Here's how the part is built. I have some questions about the finished solid (model axes, mm). A direction names the side the tool comes from. Coordinates: 2 decimals unless noted, no trailing zeros. Write each loop counter-clockwise with the first axis right and the second up, starting at its lowest first coordinate (ties: lowest second). Pieces come first, ordered by that corner, then holes.
```python
from build123d import *

# Parameters (mm, degrees)
F0_R            = 22
F1_DEPTH        = 5
F3_DEPTH        = 25
F3_COPIES_COUNT = 8
F5_DEPTH        = 8
F5_COPIES_COUNT = 4


# Not quite as in the source:
# - a pattern or mirror of a feature is missing from the dataset's text; its kind, count and spacing are read off the source's solid
# - a feature names something its author has since deleted; it is built from what else it names


with BuildPart() as f1:
    # F0 (on Front) → F1 (new body)
    with BuildSketch(Plane.XZ):
        Circle(F0_R)
    extrude(amount=F1_DEPTH)

    # F2 (on face) → F3 (cut)
    with BuildSketch(Plane.XZ.offset(5)):
        with BuildLine():
            ThreePointArc((0, -9.25), (-1.9445436483, -13.9445436483), (2.75, -12))
            ThreePointArc((2.75, -12), (1.9445436483, -10.0554563517), (0, -9.25))
        make_face()
    f3 = extrude(amount=-F3_DEPTH, mode=Mode.SUBTRACT)

    # F3_copies: F3 ×8 about axis
    f3_copies_axis = Axis((0, 0, 0), (0, 1, 0))
    for i in range(1, F3_COPIES_COUNT):
        add(f3.rotate(f3_copies_axis, i * 360 / F3_COPIES_COUNT), mode=Mode.SUBTRACT)

    # F4 (on face) → F5 (join)
    with BuildSketch(Plane(origin=(0, 0, 0), x_dir=(-1, 0, 0), z_dir=(0, 1, 0))):
        with BuildLine():
            ThreePointArc((-5.7402514855, 13.8581929877), (-4.3938929457, 14.9631208861), (-3.8883017826, 16.6298315852))
            ThreePointArc((-3.8883017826, 16.6298315852), (-9.3827106195, 18.2965422843), (-5.7402514855, 13.8581929877))
        make_face()
    f5 = extrude(amount=F5_DEPTH)

    # F5_copies: F5 ×4 about axis
    f5_copies_axis = Axis((0, 0, 0), (0, 1, 0))
    for i in range(1, F5_COPIES_COUNT):
        add(f5.rotate(f5_copies_axis, i * 360 / F5_COPIES_COUNT))


solid = f1.part
```
1) Imagine slicing it at A-A on y = 1.5. Please give me the cut outline in (x, z).
Values follow:
outline: circle Ø6 at (-16.63, 6.89); circle Ø6 at (-6.89, -16.63); circle Ø6 at (6.89, 16.63); circle Ø6 at (16.63, -6.89)
2) Will these pins go through, and if not, where does the flat tip stop? pin 1 (7 mm diameter, centred on x = 12, z = 0, fed in from -Y); pin 2 (5 mm diameter, centred on y = 0, z = 14.5, fed in from +X); pin 3 (2 mm diameter, centred on y = -1, z = 10.5, fed in from +X); pin 4 (6.5 mm diameter, centred on x = 0, z = 12, fed in from +Y).
Values follow:
pin 1: stops at y = -5
pin 2: stops at x = 18.44
pin 3: stops at x = 19.84
pin 4: stops at y = 0
3) Imagine slicing it at C-C on x = -16. Please give me the cut outline in (y, z), then the cut area to 3 significant figures.
Values follow:
outline: (-5, -15.1) - (0, -15.1) - (0, 3.96) - (8, 3.96) - (8, 9.82) - (0, 9.82) - (0, 15.1) - (-5, 15.1) - close
area: 198 mm2
4) On a 3-axis mill with a long thin cutter (end or side, diameter ignored), from which of +Z, -Z, +X, -X, +Y, -Y can I reach the whole of each face in a straight line? I mean faces 1 (the face through (0, 0, 0)), 2 (the face through (-4.769, -2.465, -21.477)). Say none if no direction works.
Values follow:
face 1: +Y
face 2: +Y, -Y
5) Imagine slicing it at B-B on x = 8. Please give me the cut outline in (y, z).
Values follow:
outline: (-5, -20.49) - (0, -20.49) - (0, -11.19) - (-5, -11.19) - close; (-5, -5.78) - (0, -5.78) - (0, 5.78) - (-5, 5.78) - close; (-5, 11.19) - (0, 11.19) - (0, 13.84) - (8, 13.84) - (8, 19.42) - (0, 19.42) - (0, 20.49) - (-5, 20.49) - close
6) Imagine slicing it at D-D on z = -18. Please give me the cut outline in (x, y).
Values follow:
outline: (-12.65, -5) - (12.65, -5) - (12.65, 0) - (-4.22, 0) - (-4.22, 8) - (-9.56, 8) - (-9.56, 0) - (-12.65, 0) - close
7) I need wall thicknesses on probe 1 along Z at (x, y) = (8, -1); probe 2 along Z at (x, y) = (-10.5, -4); probe 3 along Y at (x, z) = (10.5, 18). Which ranges of each line are inside material? Lowest first, please.
Values follow:
probe 1: z = -20.49 to -11.19, -5.78 to 5.78, 11.19 to 20.49
probe 2: z = -19.33 to -10.36, -6.61 to -2.3, 2.3 to 6.61, 10.36 to 19.33
probe 3: y = -5 to 0
